from build123d import *

# Parameters (mm, degrees)
CROQUIS1_R              = 2
SALIENTE_EXTRUIR1_DEPTH = 39
CROQUIS2_W              = 89
CROQUIS2_H              = 20
CORTAR_EXTRUIR1_DEPTH   = 39
CORTAR_EXTRUIR2_START   = -5
CROQUIS4_R              = 4
CORTAR_EXTRUIR2_DEPTH   = 24
REDONDEO1_R             = 1


with BuildPart() as part:
    # Croquis1 → Saliente-Extruir1 (new body)
    with BuildSketch(Plane.XY):
        with BuildLine():
            Line((-44.5, 6), (44.5, 6))
            ThreePointArc((44.5, 6), (50.5, 0), (44.5, -6))
            Line((44.5, -6), (-44.5, -6))
            ThreePointArc((-44.5, -6), (-50.5, 0), (-44.5, 6))
        make_face()
        with Locations((-44.5, 0)):
            Circle(CROQUIS1_R, mode=Mode.SUBTRACT)
        with Locations(Location((44.5, 0, 0), (0, 0, 180))):
            Circle(CROQUIS1_R, mode=Mode.SUBTRACT)
    extrude(amount=SALIENTE_EXTRUIR1_DEPTH)

    # Croquis2 → Cortar-Extruir1 (cut)
    with BuildSketch(Plane(origin=(0, 6, 0), x_dir=(1, 0, 0), z_dir=(0, 1, 0))):
        with Locations((0, -18.571649076)):
            Rectangle(CROQUIS2_W, CROQUIS2_H)
    extrude(amount=-CORTAR_EXTRUIR1_DEPTH, mode=Mode.SUBTRACT)

    # Croquis4 → Cortar-Extruir2 (cut)
    with BuildSketch(Plane.XY.offset(39).offset(CORTAR_EXTRUIR2_START)):
        with Locations((44.5, 0)):
            Circle(CROQUIS4_R)
        with Locations(Location((-44.5, 0, 0), (0, 0, 270))):
            Circle(CROQUIS4_R)
    extrude(amount=-CORTAR_EXTRUIR2_DEPTH, mode=Mode.SUBTRACT)

    # Redondeo1
    redondeo1_edges = [part.edges().sort_by_distance(p)[0] for p in [
        (-46.5, 0, 0),
        (46.5, 0, 0),
        (0, 6, 0),
        (50.5, 0, 0),
        (0, -6, 0),
        (-50.5, 0, 0),
    ]]
    fillet(redondeo1_edges, radius=REDONDEO1_R)


solid = part.part
Design review of the part built by this model. Coordinates are the model's own, in mm. A direction names the side the tool comes from. Coordinates: 2 decimals unless noted, no trailing zeros. Write each loop counter-clockwise with the first axis right and the second up, starting at its lowest first coordinate (ties: lowest second). Pieces come first, ordered by that corner, then holes. Notation, with made-up numbers: (61.5, -8) - (77.5, -8) arc R26 cw to (77.5, 25) - close; hole circle Ø9 at (-0.75, -15.5). An arc over 180 degrees is marked (long way). Use one line per item in the form item = value.
Q1. Insertion check: pin 1 Ø1.5 at (x, y) = (-13, -0.5) entering from -Z; pin 2 Ø1.2 at (y, z) = (-4, 23.5) entering from -X; pin 3 Ø5 at (x, y) = (-44.5, 0) entering from -Z; pin 4 Ø1 at (y, z) = (-2.5, 26) entering from -X. Each pin has a flat end and moves straight along its axis. Give the tip position at first contact, or say it passes through.
Taken from the geometry:
pin_1 = 0
pin_2 = -49.44
pin_3 = 0.13
pin_4 = -50.16
Q2. Machinability: for faces 1 (the cylindrical face through (48.315, 1.201, 24.835)), 2 (the flat face through (-1, 0, 8.572)), 3 (the cylindrical face through (-50.5, -0.1, 19.7)), which of the approach directions +Z, -Z, +X, -X, +Y, -Y give a long, thin tool a straight path to every point of the face, cutting with its end or side? Answer none if there is none.
Taken from the geometry:
face_1 = none
face_2 = +Y, -Y
face_3 = +Z, -Z, -X
Q3. Consider section D-D (z = 30). Write out the cut boundary in (x, y).
Taken from the geometry:
outline = (-44.5, -6) - (44.5, -6) arc R6 ccw to (44.5, 6) - (-44.5, 6) arc R6 ccw to start; hole circle Ø8 at (-44.5, 0); hole circle Ø8 at (44.5, 0)
Q4. The part is to be moulded in two halves that separate along Z. For faces 4 (the flat face through (-44.5, -5, 19)), 5 (the flat face through (1, -6, 34)), 6 (the flat face through (1, 0, 39)), 7 (the flat face through (1, 0, 0)), say which applies: +Z half, -Z half, draft (parallel to the pull), parting line (faces both ways), or undercut.
Taken from the geometry:
face_4 = undercut
face_5 = draft
face_6 = +Z half
face_7 = -Z half
Q5. Consider section A-A (y = 0). Count the separate pieces of the cut face and the enclosed holes in it, plus the area to 3 significant figures.
Taken from the geometry:
separate_pieces = 4
enclosed_holes = 0
area = 1,810 mm^2
Q6. Consider section C-C (x = 6.5). Write out the cut boundary in (y, z), plus the area to 3 significant figures.
Taken from the geometry:
outline = (-6, 1) arc R1 ccw to (-5, 0) - (5, 0) arc R1 ccw to (6, 1) - (6, 8.57) - (-6, 8.57) - close; (-6, 28.57) - (6, 28.57) - (6, 39) - (-6, 39) - close
area = 228 mm^2
Q7. For probe 1 along Z at (x, y) = (-6, -3); probe 2 along Y at (x, z) = (44.5, 37.55); probe 3 along Z at (x, y) = (43.5, 3.5), list the stretches that pass through material, from the lowest coordinate up.
Taken from the geometry:
probe_1 = 0 to 8.57, 28.57 to 39
probe_2 = -6 to -2, 2 to 6
probe_3 = 0 to 8.57, 34 to 39
Q8. Consider section B-B (z = 14.5). Write out the cut boundary in (x, y), plus the area to 3 significant figures.
Taken from the geometry:
outline = (-44.5, -6) - (-44.5, -4) arc R4 cw to (-44.5, 4) - (-44.5, 6) arc R6 ccw to start; (44.5, -6) arc R6 ccw to (44.5, 6) - (44.5, 4) arc R4 cw to (44.5, -4) - close
area = 62.8 mm^2
